Read the model definition and answer for the solid it produces. Units are mm, in the model's axes. A direction names the side the tool comes from. Coordinates: 2 decimals unless noted, no trailing zeros. Write each loop counter-clockwise with the first axis right and the second up, starting at its lowest first coordinate (ties: lowest second). Pieces come first, ordered by that corner, then holes.
(1) Given pin 1 (15 mm diameter, centred on y = 26, z = 6, fed in from +X); pin 2 (1.5 mm diameter, centred on x = -37.5, z = 18.5, fed in from -Y); pin 3 (4 mm diameter, centred on x = 4, y = 32, fed in from +Z), each flat-ended and moving along its own axis, determine where each tip first touches the part or whether it passes through.
(2) Which of the six approach directions +Z, -Z, +X, -X, +Y, -Y give full straight-line access (tool end or side, diameter ignored) to faces 4 (the cylindrical face through (-23.406, 16.887, 48.224)), 5 (the flat face through (-2.546, 33, 7)), 6 (the flat face through (4, 29, 13.669)), 7 (the flat face through (-18, -25, 0)), 8 (the flat face through (-51.343, -34, 25))?
(3) Find the intervals of material crossed by probe 1 along X at (y, z) = (28.5, 3); probe 2 along Z at (x, y) = (-14.5, 8.5); probe 3 along X at (y, z) = (35, 5), in increasing order.
(4) Section A-A on z = 33.5 is taken. Write down the section's boundary in (x, y).
(5) Section C-C on y = 18 is taken. Write down the section's boundary in (x, z).
(6) The mould has two halves that part along Y. Classify faces 1 (the flat face through (10.269, 25, 7)), 2 (the flat face through (-33.7, 21.765, 25.044)), 3 (the flat face through (4, -48, 5.08)): +Y half, -Y half, draft (parallel to the pull), parting line (faces both ways), or undercut.
(7) Section D-D on x = -15 is taken. Write down the section's boundary in (y, z), then the cut area to 3 significant figures.
(8) Section B-B on y = 35 is taken. Write down the section's boundary in (x, z), then the cut area to 3 significant figures.
from build123d import *

# Parameters (mm, degrees)
F0_R     = 9.3096662381
F1_DEPTH = 50.8
F2_DEPTH = 13.66946
F3_DEPTH = 45.83504
F4_START = 5.08
F4_DEPTH = 40.64
F5_START = 5.08
F5_DEPTH = 40.64


with BuildPart() as f1:
    # F0 (on Top) → F1 (new body)
    with BuildSketch(Plane.XY):
        Polygon((-51.3433143497, 0), (-51.3433143497, -69.4561004639), (-32.0200270793, -69.294249187), (-32.3172560351, -33.8083351523), (-11.77348243, -33.6362611184), (-11.4762534741, -69.122175153), (16.7662296444, -68.8856169581), (16.7662296444, 0), (10.2686649188, 8.3737781411), (-2.5458205626, 24.8885283509), (-16.5439583361, 42.9287180305), align=None)
        Polygon((-3.6103976934, -57.465070353), (-3.772769589, -38.0796268582), (12.3200837265, -38.0858059556), (12.4812749246, -57.3302869839), align=None, mode=Mode.SUBTRACT)
        with Locations((-16.5439583361, 10.5952649524)):
            Circle(F0_R, mode=Mode.SUBTRACT)
    extrude(amount=F1_DEPTH)

    # F0 (on Top) → F2 (join)
    with BuildSketch(Plane.XY):
        Polygon((-2.5458205626, 41.5025129914), (-2.5458205626, 24.8885283509), (10.2686649188, 8.3737781411), (10.2686649188, 41.5025129914), align=None)
    extrude(amount=F2_DEPTH)

    # F0 (on Top) → F3 (join)
    with BuildSketch(Plane.XY):
        Polygon((-32.3172560351, -33.8083351523), (-32.0200270793, -69.294249187), (-11.4762534741, -69.122175153), (-11.77348243, -33.6362611184), align=None)
    extrude(amount=F3_DEPTH)

    # F0 (on Top) → F4 (join)
    with BuildSketch(Plane.XY.offset(F4_START)):
        Polygon((12.3200837265, -38.0858059556), (-3.772769589, -38.0796268582), (-3.6103976934, -57.465070353), (12.4812749246, -57.3302869839), align=None)
    extrude(amount=F4_DEPTH)

    # F0 (on Top) → F5 (join)
    with BuildSketch(Plane.XY.offset(F5_START)):
        with Locations((-16.5439583361, 10.5952649524)):
            Circle(F0_R)
    extrude(amount=F5_DEPTH)


solid = f1.part
Response:
1. pin 1: stops at x = 10.27
1. pin 2: stops at y = -69.35
1. pin 3: stops at z = 13.67
2. face 4: +Z
2. face 5: +Z, -Z, +Y
2. face 6: +Z, +X, +Y
2. face 7: -Z, +X, -X, +Y, -Y
2. face 8: +Z, -Z, -X, +Y, -Y
3. probe 1: x = -28.24 to -5.35, -2.55 to 10.27
3. probe 2: z = 5.08 to 45.72
3. probe 3: x = -22.97 to -10.39, -2.55 to 10.27
4. outline: (-51.34, -69.46) - (16.77, -68.89) - (16.77, 0) - (-16.54, 42.93) - (-51.34, 0) - close
5. outline: (-36.75, 0) - (-22.19, 0) - (-22.19, 5.08) - (-10.9, 5.08) - (-10.9, 0) - (10.27, 0) - (10.27, 13.67) - (2.8, 13.67) - (2.8, 50.8) - (-10.9, 50.8) - (-10.9, 45.72) - (-22.19, 45.72) - (-22.19, 50.8) - (-36.75, 50.8) - close
6. face 1: draft
6. face 2: +Y half
6. face 3: undercut
7. outline: (-69.15, 0) - (1.41, 0) - (1.41, 5.08) - (19.78, 5.08) - (19.78, 0) - (40.94, 0) - (40.94, 50.8) - (19.78, 50.8) - (19.78, 45.72) - (1.41, 45.72) - (1.41, 50.8) - (-33.66, 50.8) - (-33.66, 45.84) - (-69.15, 45.84) - close
7. area: 5,230 mm2
8. outline: (-22.97, 0) - (-10.39, 0) - (-10.39, 50.8) - (-22.97, 50.8) - close; (-2.55, 0) - (10.27, 0) - (10.27, 13.67) - (-2.55, 13.67) - close
8. area: 814 mm2
